Can you work these out from the model? Positions are in its coordinate system, mm. Face numbers are marked on the shaded views. Give positions to 0.01 mm unless a question says otherwise; leave off trailing zeros. Order: outer loops, then holes, each group sorted by start corner. A loop starts at its lowest first (then second) coordinate and runs counter-clockwise, first axis right, second up. Notation, with made-up numbers: (21, -28.5) - (58, -28.5) arc R14 cw to (58, -7.5) - close; hole circle Ø2 at (41, 41.5). An arc over 180 degrees is marked (long way). Answer as a JSON object with one key per item and string values.
```python
from build123d import *

# Parameters (mm, degrees)
F0_W         = 35
F0_H         = 35
F1_DEPTH     = 6.5
F2_R         = 2.125
F3_DEPTH     = 13.001
F4_R         = 5
F5_T1_DEPTH  = 25
F5_T3_DEPTH  = 25
F5_T12_ANGLE = 90
F5_T14_ANGLE = 90
F5_T16_ANGLE = 90
F5_T18_ANGLE = 90
F6_R         = 4
F7_DEPTH     = 13.001
F8_SIZE      = 1


# Not quite as in the source:
# - a fillet or chamfer that OpenCascade refuses, or shapes differently, is made with other operations: its cross-section is extruded or revolved along the edge and cut away or added


with BuildPart() as f1:
    # F0 (on Top) → F1 (new body, symmetric)
    with BuildSketch(Plane.XY):
        Rectangle(F0_W, F0_H)
    extrude(amount=F1_DEPTH, both=True)

    # F2 (on face) → F3 (cut, through all)
    with BuildSketch(Plane.XY.offset(6.5)):
        with Locations((-12.5, -12.9)):
            Circle(F2_R)
        with Locations((-12.5, 12.5)):
            Circle(F2_R)
        with Locations((12.5, 12.5)):
            Circle(F2_R)
        with Locations((12.5, -12.9)):
            Circle(F2_R)
    extrude(amount=-F3_DEPTH, mode=Mode.SUBTRACT)

    # F4
    f4_edges = [f1.edges().sort_by_distance(p)[0] for p in [
        (-17.5, 17.5, 0),
        (17.5, 17.5, 0),
        (17.5, -17.5, 0),
        (-17.5, -17.5, 0),
    ]]
    fillet(f4_edges, radius=F4_R)

    # F5: chamfer of 1.4 x 2.8 on 12 edges, made by hand

    # F5_s2 → F5_t1 (cut)
    with BuildSketch(Plane.XZ.offset(-12.5)):
        Polygon((17.5, -3.7), (16.1, -6.5), (17.5, -6.5), align=None)
        Polygon((-16.1, -6.5), (-17.5, -3.7), (-17.5, -6.5), align=None)
    extrude(amount=F5_T1_DEPTH, mode=Mode.SUBTRACT)

    # F5_s4 → F5_t3 (cut)
    with BuildSketch(Plane.YZ.offset(-12.5)):
        Polygon((-16.1, -6.5), (-17.5, -3.7), (-17.5, -6.5), align=None)
        Polygon((16.1, -6.5), (17.5, -3.7), (17.5, -6.5), align=None)
    extrude(amount=F5_T3_DEPTH, mode=Mode.SUBTRACT)

    # F5_s5 → F5_t6 (revolve, cut)
    with BuildSketch(Plane.XZ.offset(12.9)):
        Polygon((-8.975, -6.5), (-10.375, -3.7), (-10.375, -6.5), align=None)
    revolve(axis=Axis((-12.5, -12.9, -6.5), (0, 0, 1)), mode=Mode.SUBTRACT)

    # F5_s7 → F5_t8 (revolve, cut)
    with BuildSketch(Plane.XZ.offset(12.9)):
        Polygon((16.025, -6.5), (14.625, -3.7), (14.625, -6.5), align=None)
    revolve(axis=Axis((12.5, -12.9, -6.5), (0, 0, 1)), mode=Mode.SUBTRACT)

    # F5_s9 → F5_t10 (revolve, cut)
    with BuildSketch(Plane.XZ.offset(-12.5)):
        Polygon((16.025, -6.5), (14.625, -3.7), (14.625, -6.5), align=None)
    revolve(axis=Axis((12.5, 12.5, -6.5), (0, 0, 1)), mode=Mode.SUBTRACT)

    # F5_s11 → F5_t12 (revolve, cut)
    with BuildSketch(Plane.XZ.offset(12.5)):
        Polygon((16.1, -6.5), (17.5, -3.7), (17.5, -6.5), align=None)
    revolve(axis=Axis((12.5, -12.5, -6.5), (0, 0, -1)), revolution_arc=F5_T12_ANGLE, mode=Mode.SUBTRACT)

    # F5_s13 → F5_t14 (revolve, cut)
    with BuildSketch(Plane.XZ.offset(-12.5)):
        Polygon((16.1, -6.5), (17.5, -3.7), (17.5, -6.5), align=None)
    revolve(axis=Axis((12.5, 12.5, -6.5), (0, 0, 1)), revolution_arc=F5_T14_ANGLE, mode=Mode.SUBTRACT)

    # F5_s15 → F5_t16 (revolve, cut)
    with BuildSketch(Plane.YZ.offset(-12.5)):
        Polygon((-16.1, -6.5), (-17.5, -3.7), (-17.5, -6.5), align=None)
    revolve(axis=Axis((-12.5, -12.5, -6.5), (0, 0, -1)), revolution_arc=F5_T16_ANGLE, mode=Mode.SUBTRACT)

    # F5_s17 → F5_t18 (revolve, cut)
    with BuildSketch(Plane.YZ.offset(-12.5)):
        Polygon((16.1, -6.5), (17.5, -3.7), (17.5, -6.5), align=None)
    revolve(axis=Axis((-12.5, 12.5, -6.5), (0, 0, 1)), revolution_arc=F5_T18_ANGLE, mode=Mode.SUBTRACT)

    # F5_s19 → F5_t20 (revolve, cut)
    with BuildSketch(Plane.XZ.offset(-12.5)):
        Polygon((-8.975, -6.5), (-10.375, -3.7), (-10.375, -6.5), align=None)
    revolve(axis=Axis((-12.5, 12.5, -6.5), (0, 0, 1)), mode=Mode.SUBTRACT)

    # F6 (on face) → F7 (cut, through all)
    with BuildSketch(Plane(origin=(0, 0, -6.5), x_dir=(1, 0, 0), z_dir=(0, 0, -1))):
        Circle(F6_R)
    extrude(amount=-F7_DEPTH, mode=Mode.SUBTRACT)

    # F8
    f8_edges = [f1.edges().sort_by_distance(p)[0] for p in [
        (-16.035534, -16.035534, 6.5),
    ]]
    chamfer(f8_edges, length=F8_SIZE)


solid = f1.part
```
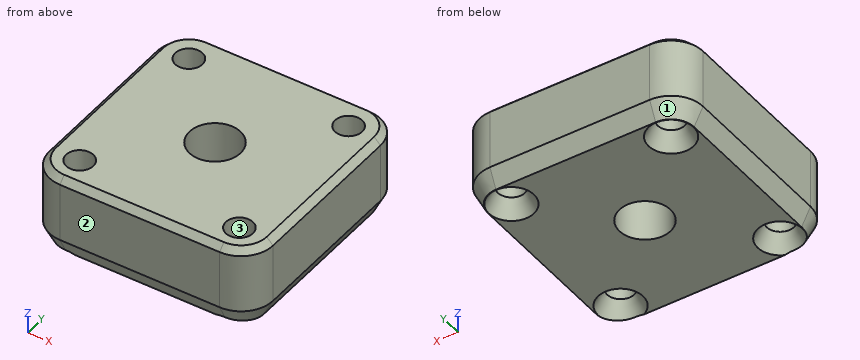
Q1. If we section it at A-A, the plane z = 0.25: Please give me the cut outline in (x, y) (3 decimals), then the cut area to 3 significant figures.
Recorded:
{"outline": "(-17.5, -12.5) arc R5 ccw to (-12.5, -17.5) - (12.5, -17.5) arc R5 ccw to (17.5, -12.5) - (17.5, 12.5) arc R5 ccw to (12.5, 17.5) - (-12.5, 17.5) arc R5 ccw to (-17.5, 12.5) - close; hole circle Ø4.25 at (-12.5, -12.9); hole circle Ø4.25 at (-12.5, 12.5); hole circle Ø8 at (0, 0); hole circle Ø4.25 at (12.5, -12.9); hole circle Ø4.25 at (12.5, 12.5)", "area": "1,100 mm^2"}
Q2. If we section it at D-D, the plane z = -5.5: Please give me the cut outline in (x, y) (3 decimals), then the cut area to 3 significant figures.
Recorded:
{"outline": "(-16.6, -12.5) arc R4.1 ccw to (-12.5, -16.6) - (12.5, -16.6) arc R4.1 ccw to (16.6, -12.5) - (16.6, 12.5) arc R4.1 ccw to (12.5, 16.6) - (-12.5, 16.6) arc R4.1 ccw to (-16.6, 12.5) - close; hole circle Ø6.05 at (-12.5, -12.9); hole circle Ø6.05 at (-12.5, 12.5); hole circle Ø8 at (0, 0); hole circle Ø6.05 at (12.5, -12.9); hole circle Ø6.05 at (12.5, 12.5)", "area": "923 mm^2"}
Q3. I need wall thicknesses on L1, parallel to Y at x = 12.5, z = -1 (3 decimals); L2, parallel to Y at x = 0, z = 2.25; L3, parallel to Y at x = -11, z = -3. Which ranges of each line are inside material? Lowest first, please.
Recorded:
{"L1": "y = -17.5 to -15.025, -10.775 to 10.375, 14.625 to 17.5", "L2": "y = -17.5 to -4, 4 to 17.5", "L3": "y = -17.5 to -14.41, -11.39 to 10.99, 14.01 to 17.5"}
Q4. We'd pull the mould along Y, two halves only. Please class the marked faces 1, 2 and 3: released by +Y, released by -Y, zero draft, split by the parting line, or undercut.
Recorded:
{"face 1": "released by +Y", "face 2": "released by -Y", "face 3": "undercut"}
Q5. If we section it at B-B, the plane y = 0: Please give me the cut outline in (x, z), then the cut area to 3 significant figures.
Recorded:
{"outline": "(-17.5, -3.7) - (-16.1, -6.5) - (-4, -6.5) - (-4, 6.5) - (-16.5, 6.5) - (-17.5, 5.5) - close; (4, -6.5) - (16.1, -6.5) - (17.5, -3.7) - (17.5, 5.5) - (16.5, 6.5) - (4, 6.5) - close", "area": "346 mm^2"}
